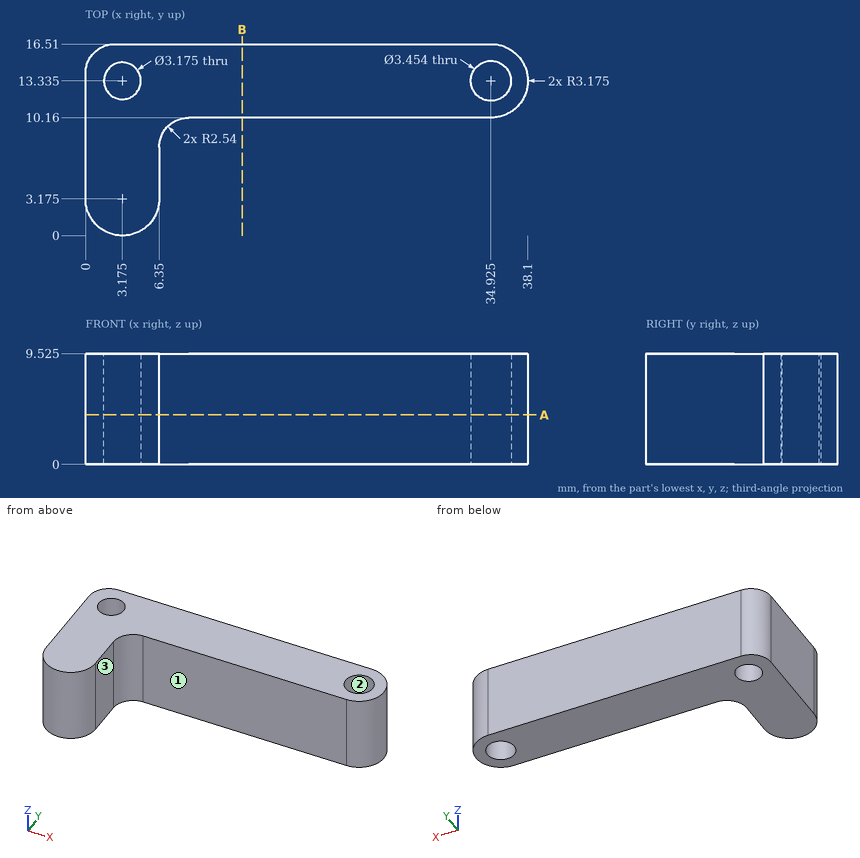
Input: dimensioned drawing with shaded views. Units: mm. Origin: part minimum x, y, z. Coordinates: 2 decimals unless noted, no trailing zeros. Order: outer loops, then holes, each group sorted by start corner. A loop starts at its lowest first (then second) coordinate and runs counter-clockwise, first axis right, second up. Notation, with made-up numbers: (79.25, 66) - (118.25, 66) arc R22 ccw to (118.25, 94) - close; hole circle Ø9 at (31, 77.5). An arc over 180 degrees is marked (long way). Put each result on its own line as item: value.
1. Draft query along X for the marked faces 1, 2 and 3. Return one class per face: pulls with the +X half, pulls with the -X half, needs draft (parallel to the pull), parting line crosses it, or undercut.
Report:
face 1: needs draft
face 2: undercut
face 3: pulls with the +X half
2. Contact query for flat-ended pins moving along their axis: pin 1 Ø2 at (x, z) = (22, 1.5) entering from -Y; pin 2 Ø2 at (y, z) = (5, 3) entering from +X; pin 3 Ø1 at (y, z) = (8, 8.5) entering from +X; pin 4 Ø2.5 at (x, y) = (3.175, 13.335) entering from +Z. Output: stop coordinate, or through.
Report:
pin 1: stops at y = 10.16
pin 2: stops at x = 6.35
pin 3: stops at x = 6.51
pin 4: passes through
3. Line query: line 1 along X through (y, z) = (12, 0.5) (1 decimal); line 2 along Y through (x, z) = (32.5, 1.75); line 3 along X through (y, z) = (12.25, 1) (1 decimal). Output: solid intervals per line, ascending.
Report:
line 1: x = 0 to 2.3, 4 to 33.8, 36 to 37.8
line 2: y = 10.16 to 16.51
line 3: x = 0 to 2, 4.3 to 33.6, 36.3 to 37.9
4. Cut plane B-B on x = 13.5. Return the cut outline in (y, z) (1 decimal).
Report:
outline: (10.2, 0) - (16.5, 0) - (16.5, 9.5) - (10.2, 9.5) - close
5. Cut plane A-A on z = 4.25. State how many separate pieces and enclosed holes the cut face has.
Report:
separate pieces: 1
enclosed holes: 2
